from build123d import *

# Parameters (mm, degrees)
ESQUISSE1_R        = 45
BOSS_EXTRU_1_DEPTH = 700
ESQUISSE2_R        = 40
BOSS_EXTRU_4_DEPTH = 700
ESQUISSE3_R        = 35
BOSS_EXTRU_5_DEPTH = 700
ESQUISSE4_R        = 30
BOSS_EXTRU_6_DEPTH = 700
BOSS_EXTRU_7_DEPTH = 60


with BuildPart() as part:
    # Esquisse1 → Boss.-Extru.1 (new body)
    with BuildSketch(Plane.XY):
        with Locations((-5.0559795, 0.208317709)):
            Circle(ESQUISSE1_R)
    extrude(amount=BOSS_EXTRU_1_DEPTH)

    # Esquisse2 → Boss.-Extru.4 (add)
    with BuildSketch(Plane(origin=(0, 0, 0), x_dir=(-1, 0, 0), z_dir=(0, 0, -1))):
        with Locations(Location((5.0559795, 0.208317709, 0), (0, 0, 180))):
            Circle(ESQUISSE2_R)
    extrude(amount=BOSS_EXTRU_4_DEPTH)

    # Esquisse3 → Boss.-Extru.5 (add)
    with BuildSketch(Plane(origin=(0, 0, -700), x_dir=(-1, 0, 0), z_dir=(0, 0, -1))):
        with Locations((5.0559795, 0.208317709)):
            Circle(ESQUISSE3_R)
    extrude(amount=BOSS_EXTRU_5_DEPTH)

    # Esquisse4 → Boss.-Extru.6 (add)
    with BuildSketch(Plane(origin=(0, 0, -1400), x_dir=(-1, 0, 0), z_dir=(0, 0, -1))):
        with Locations((5.0559795, 0.208317709)):
            Circle(ESQUISSE4_R)
    extrude(amount=BOSS_EXTRU_6_DEPTH)

    # Esquisse5 → Boss.-Extru.7 (add)
    with BuildSketch(Plane(origin=(0, 0, -2100), x_dir=(-1, 0, 0), z_dir=(0, 0, -1))):
        Polygon((4.785922621, -107.572959404), (112.836533333, -0.270056879), (5.305557146, 108.010216758), (-102.745053566, 0.707314234), align=None)
    extrude(amount=BOSS_EXTRU_7_DEPTH)


solid = part.part
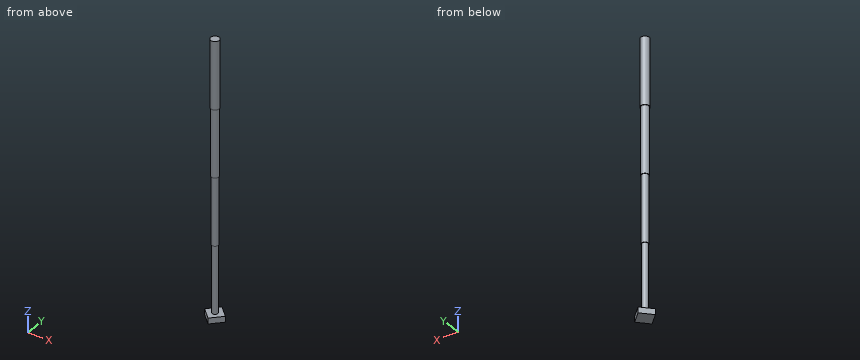
Work out the finished part from the listing and answer in its coordinate system (mm). Coordinates: 2 decimals unless noted, no trailing zeros. Write each loop counter-clockwise with the first axis right and the second up, starting at its lowest first coordinate (ties: lowest second). Pieces come first, ordered by that corner, then holes. Notation, with made-up numbers: M 86,20.25 L 113,20.25 A37 ccw 113,58.25 Z; hole C -17.5,25 d2. An arc over 180 degrees is marked long. Use one line per item in the form item = value. Start each with the question number.
1. Straight lines are drawn through the part: probe 1 along Z at (x, y) = (-5.5, -41); probe 2 along Z at (x, y) = (62, 2.5); probe 3 along X at (y, z) = (-1, -1502). For each, find the intervals that lie inside material, in ascending order. Write a range as from..to.
2. Each of these flat-tipped pins is pushed along its axis until it touches: P1, Ø12, axis at y = 4, z = -94.5, coming from the +X side; P2, Ø10, axis at y = -15.5, z = -1214, coming from the -X side; P3, Ø1, axis at y = 33.5, z = 355.5, coming from the +X side. Where does it stop, or does it pass through?
3. The part is cut by section C-C (z = -1017). Give the vertices of the cut face in (x, y).
4. The part is cut by section B-B (y = -69.5). Give the vertices of the cut face in (x, z), plus the area to 3 significant figures.
5. The part is cut by section A-A (z = -1676). Give the vertices of the cut face in (x, y), plus the area to 3 significant figures.
Evaluation:
q1.probe_1 = -2160..-2100, 0..700
q1.probe_2 = -2160..-2100
q1.probe_3 = -35.03..24.92
q2.P1 = 34.94
q2.P2 = -38.38
q2.P3 = 25.76
q3.outline = C -5.06,0.21 d70
q4.outline = M -43.12,-2160 L 33.02,-2160 L 33.02,-2100 L -43.12,-2100 Z
q4.area = 4,570 mm^2
q5.outline = C -5.06,0.21 d60
q5.area = 2,830 mm^2
